```python
from build123d import *

# Parameters (mm, degrees)
SKETCH_5_W          = 10
SKETCH_5_H          = 30
EXTRUDE_5_DEPTH     = 3
SKETCH_6_W          = 30
SKETCH_6_H          = 100
SKETCH_6_H_2        = 3
EXTRUDE_6_DEPTH     = 3
CUT_EXTRUDE_2_DEPTH = 3


with BuildPart() as part:
    # 草图5 → 凸台-拉伸5 (new body)
    with BuildSketch(Plane(origin=(0, 0, 0), x_dir=(1, 0, 0), z_dir=(0, 1, 0))):
        with Locations((5, -15)):
            Rectangle(SKETCH_5_W, SKETCH_5_H)
        with BuildLine():
            Line((8, -5), (8, -25))
            ThreePointArc((8, -25), (5, -28), (2, -25))
            Line((2, -25), (2, -5))
            ThreePointArc((2, -5), (5, -2), (8, -5))
        make_face(mode=Mode.SUBTRACT)
    extrude(amount=EXTRUDE_5_DEPTH)

    # 草图6 → 凸台-拉伸6 (add)
    with BuildSketch(Plane(origin=(10, 0, 0), x_dir=(0, 0, -1), z_dir=(1, 0, 0))):
        with Locations((-15, 53)):
            Rectangle(SKETCH_6_W, SKETCH_6_H)
        with Locations((-15, 1.5)):
            Rectangle(SKETCH_6_W, SKETCH_6_H_2)
    extrude(amount=EXTRUDE_6_DEPTH)

    # 草图7 → 切除-拉伸2 (cut)
    with BuildSketch(Plane.ZY.offset(-10)):
        with BuildLine():
            Line((16.5, 90), (16.5, 20))
            ThreePointArc((16.5, 20), (15, 18.5), (13.5, 20))
            Line((13.5, 20), (13.5, 90))
            ThreePointArc((13.5, 90), (15, 91.5), (16.5, 90))
        make_face()
    extrude(amount=-CUT_EXTRUDE_2_DEPTH, mode=Mode.SUBTRACT)


solid = part.part
```
Can you work these out from the model? Positions are in its coordinate system, mm. A direction names the side the tool comes from. Round coordinates to 2 decimals unless told otherwise and drop trailing zeros. Loops run counter-clockwise (first coordinate to the right, second up) from the corner with the lowest first, then second, coordinate; pieces in that order, holes last. Notation, with made-up numbers: M 14,5 L 50,5 A17 ccw 50,35 Z; hole C 41,81 d8. An arc over 180 degrees is marked long. Write item = value, one per line. Start each with the question number.
(1) Suppose I cut it at C-C on x = 11. Write out the boundary of the cut face in (y, z).
(2) If we mould it in two halves opening along Y, with no side actions, what happens to faces 1 (the face through (11, 55, 16.5)), 2 (the face through (10, 54, 19)), 3 (the face through (9, 0, 15))? For each: released by +Y, released by -Y, zero draft, split by the parting line, or undercut.
(3) Suppose I cut it at B-B on y = 47. Write out the boundary of the cut face in (x, z), plus the area to 3 significant figures.
(4) Which directions (+Z, -Z, +X, -X, +Y, -Y) give clear straight access to the entire face, cutting with the end or side of a thin tool? Please do faces 4 (the face through (1.6, 3, 14.8)), 5 (the face through (11.5, 91.5, 15)), 6 (the face through (13, 52, 19)), 7 (the face through (5, 1, 2)).
(5) I'm going to push flat-ended pins straight in: P1, Ø12, axis at y = 47.5, z = 16.5, coming from the -X side; P2, Ø1, axis at x = 4, z = 5, coming from the -Y side. Where does each tip first touch, or does it pass through?
(6) Suppose I cut it at A-A on z = 15. Write out the boundary of the cut face in (x, y).
(7) I need wall thicknesses on line 1 along Z through (x, y) = (12.25, 35.5); line 2 along Y through (x, z) = (9, 22); line 3 along X through (y, z) = (33.5, 11.75). Which ranges of each line are inside material? Lowest first, please.
Answer block:
q1.outline = M 0,0 L 103,0 L 103,30 L 0,30 Z; hole M 20,13.5 L 90,13.5 A1.5 ccw 90,16.5 L 20,16.5 A1.5 ccw Z
q2.face_1 = undercut
q2.face_2 = zero draft
q2.face_3 = released by -Y
q3.outline = M 10,0 L 13,0 L 13,13.5 L 10,13.5 Z; M 10,16.5 L 13,16.5 L 13,30 L 10,30 Z
q3.area = 81.0 mm²
q4.face_4 = +Z, -Z, -X, +Y
q4.face_5 = +X, -X
q4.face_6 = +Z, -Z, +X, +Y, -Y
q4.face_7 = +Y, -Y
q5.P1 = 10
q5.P2 = through
q6.outline = M 0,0 L 2,0 L 2,3 L 0,3 Z; M 8,0 L 13,0 L 13,18.5 L 10,18.5 L 10,3 L 8,3 Z; M 10,91.5 L 13,91.5 L 13,103 L 10,103 Z
q7.line_1 = 0 to 13.5, 16.5 to 30
q7.line_2 = 0 to 3
q7.line_3 = 10 to 13
